The drawing under review shows one solid part. Ordinate dimensions are in mm from its lowest x, y, z. A direction names the side the tool comes from. Round coordinates to 2 decimals unless told otherwise and drop trailing zeros. Order: outer loops, then holes, each group sorted by start corner. A loop starts at its lowest first (then second) coordinate and runs counter-clockwise, first axis right, second up. Notation, with made-up numbers: (12, 16) -> (65, 16) arc R10 cw to (65, 27) -> close; hole circle Ø4 at (35, 88). An arc over 180 degrees is marked (long way). Use a Markdown table: item, result. Add a question column.
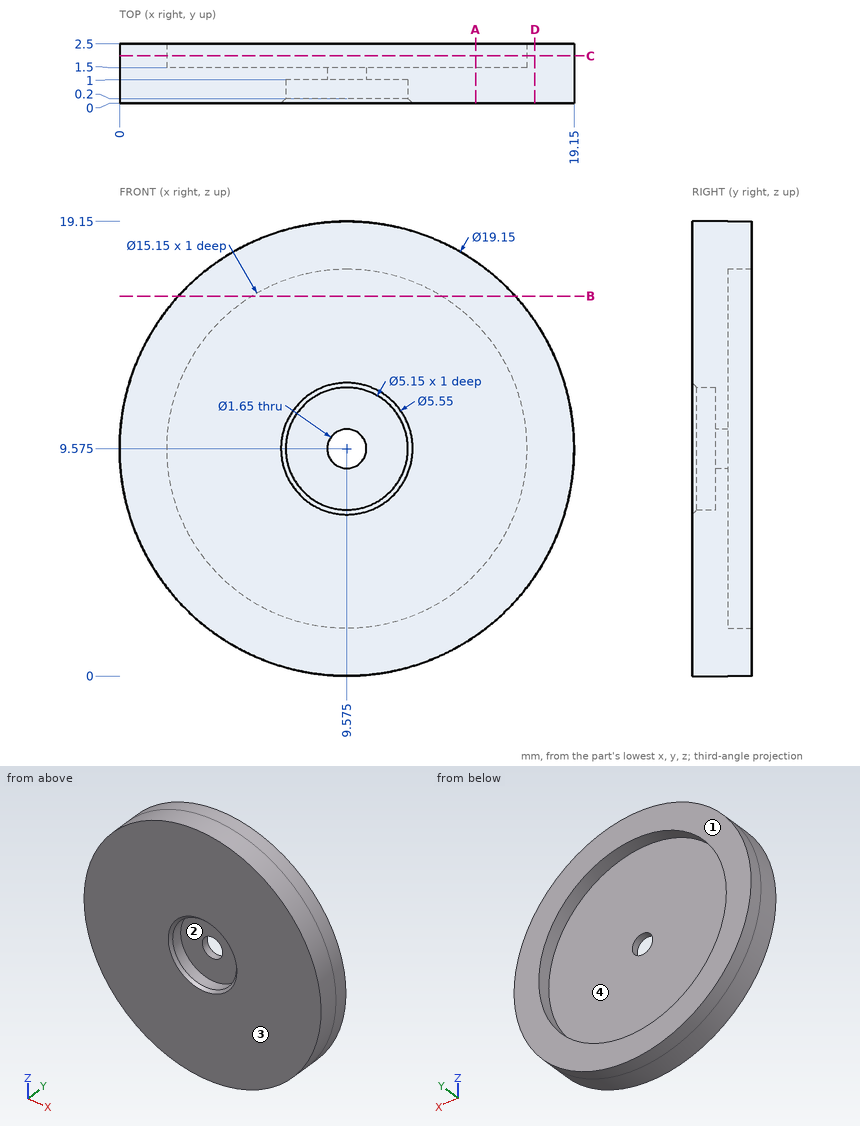
Q1. For the marked faces 3 and 4, list the 3-axis set-ups (+Z, -Z, +X, -X, +Y, -Y) from which the entire face can be reached by the end or side of a thin tool; tool diameter is ignored.
Q2. Draft analysis for pull direction X (two halves, no side actions). For the marked faces 1 and 2, state which applies: released by +X, released by -X, zero draft, split by the parting line, or undercut.
Q3. Add section B-B, the plane z = 16. Give the boundary of the cut face in (x, y), then the cut area to 3 significant figures.
Q4. Add section A-A, the plane x = 15. Give the boundary of the cut face in (y, z), then the cut area to 3 significant figures.
Q5. Add section C-C, the plane y = 2. Give the boundary of the cut face in (x, z) (3 decimals).
Q6. Add section D-D, the plane x = 17.5. Give the boundary of the cut face in (y, z), then the cut area to 3 significant figures.
Q7. To check wall thickness, follow line 1 along Z through (x, y) = (9.75, 0.25); line 2 along Y through (x, z) = (8, 11.5); line 3 along Y through (x, z) = (15.75, 13). State the ranges of each line that lie inside material, in increasing order.
Q8. For pin 1 (4.5 mm diameter, centred on x = 9.575, z = 9.575, fed in from +Y); pin 2 (1.5 mm diameter, centred on x = 10.5, z = 10.5, fed in from -Y); pin 3 (1.3 mm diameter, centred on x = 9.575, z = 9.575, fed in from -Y); pin 4 (1 mm diameter, centred on x = 10.5, y = 1.5, fed in from +Z), all flat-tipped, find the tip position at first contact; note any pin that passes through.
Return value:
| question | item | result |
|---|---|---|
| 1 | face 3 | +Z, -Z, +X, -X, -Y |
| 1 | face 4 | +Y |
| 2 | face 1 | zero draft |
| 2 | face 2 | undercut |
| 3 | outline | (2.48, 0) -> (16.67, 0) -> (16.67, 2.5) -> (13.59, 2.5) -> (13.59, 1.5) -> (5.56, 1.5) -> (5.56, 2.5) -> (2.48, 2.5) -> close |
| 3 | area | 27.5 mm² |
| 4 | outline | (0, 1.69) -> (2.5, 1.69) -> (2.5, 4.29) -> (1.5, 4.29) -> (1.5, 14.86) -> (2.5, 14.86) -> (2.5, 17.46) -> (0, 17.46) -> close |
| 4 | area | 28.9 mm² |
| 5 | outline | circle Ø19.15 at (9.575, 9.575); hole circle Ø15.15 at (9.575, 9.575) |
| 6 | outline | (0, 4.2) -> (2.5, 4.2) -> (2.5, 14.95) -> (0, 14.95) -> close |
| 6 | area | 26.9 mm² |
| 7 | line 1 | 0 to 7.01, 12.14 to 19.15 |
| 7 | line 2 | 1 to 1.5 |
| 7 | line 3 | 0 to 1.5 |
| 8 | pin 1 | y = 1.5 |
| 8 | pin 2 | y = 1 |
| 8 | pin 3 | through |
| 8 | pin 4 | z = 19.14 |
